```python
from build123d import *

# Parameters (mm, degrees)
F0_R     = 30.180652
F1_DEPTH = 254
F2_R     = 23.830652
F3_DEPTH = 102.916548
F4_R     = 5.08
F6_W     = 42.340428
F6_H     = 35.694406
F7_DEPTH = 45.834139


with BuildPart() as f1:
    # F0 (on Top) → F1 (new body)
    with BuildSketch(Plane.XY):
        Circle(F0_R)
    extrude(amount=-F1_DEPTH)

    # F2 (on face) → F3 (cut)
    with BuildSketch(Plane(origin=(0, 0, -254), x_dir=(1, 0, 0), z_dir=(0, 0, -1))):
        Circle(F2_R)
    extrude(amount=-F3_DEPTH, mode=Mode.SUBTRACT)

    # F4
    f4_edges = [f1.edges().sort_by_distance(p)[0] for p in [
        (30.180652, 0, -127),
        (-30.180652, 0, 0),
        (-30.180652, 0, -254),
    ]]
    fillet(f4_edges, radius=F4_R)

    # F6 (on offset) → F7 (join)
    with BuildSketch(Plane.YZ.offset(55.124739)):
        with Locations((3.907934, -50.849177)):
            Rectangle(F6_W, F6_H)
    extrude(amount=-F7_DEPTH)


solid = f1.part
```
For this review, take the finished solid that the model builds, in its own axes (mm). A direction names the side the tool comes from. Round coordinates to 2 decimals unless told otherwise and drop trailing zeros. Write each loop counter-clockwise with the first axis right and the second up, starting at its lowest first coordinate (ties: lowest second). Pieces come first, ordered by that corner, then holes.
1) Take a section at B-B on y = 0. Give the boundary of the cut face in (x, z), then the cut area to 3 significant figures.
Answer below:
outline: (-30.18, -248.92) arc R5.08 ccw to (-25.1, -254) - (-23.83, -254) - (-23.83, -151.08) - (23.83, -151.08) - (23.83, -254) - (25.1, -254) arc R5.08 ccw to (30.18, -248.92) - (30.18, -68.7) - (55.12, -68.7) - (55.12, -33) - (30.18, -33) - (30.18, -5.08) arc R5.08 ccw to (25.1, 0) - (-25.1, 0) arc R5.08 ccw to (-30.18, -5.08) - close
area: 11,300 mm2
2) For line 1 along Y through (x, z) = (0, -228); line 2 along Z through (x, y) = (12.5, -9); line 3 along Y through (x, z) = (2.5, -242.5), list the stretches that pass through material, from the lowest coordinate up.
Answer below:
line 1: y = -30.18 to -23.83, 23.83 to 30.18
line 2: z = -151.08 to 0
line 3: y = -30.08 to -23.7, 23.7 to 30.08
3) Take a section at A-A on x = 0. Give the boundary of the cut face in (y, z), then the cut area to 3 significant figures.
Answer below:
outline: (-30.18, -248.92) arc R5.08 ccw to (-25.1, -254) - (-23.83, -254) - (-23.83, -151.08) - (23.83, -151.08) - (23.83, -254) - (25.1, -254) arc R5.08 ccw to (30.18, -248.92) - (30.18, -5.08) arc R5.08 ccw to (25.1, 0) - (-25.1, 0) arc R5.08 ccw to (-30.18, -5.08) - close
area: 10,400 mm2
4) Machinability: for faces 1 (the face through (12.8, -20.1, -203.3)), 2 (the face through (22.2, -9.2, -254)), 3 (the face through (40, -17.262, -51)), which of the approach directions +Z, -Z, +X, -X, +Y, -Y give a long, thin tool a straight path to every point of the face, cutting with its end or side? Answer none if there is none.
Answer below:
face 1: -Z
face 2: -Z, +X, -X, +Y, -Y
face 3: +Z, -Z, +X, -Y
5) Take a section at D-D on x = 40. Give the boundary of the cut face in (y, z), then the cut area to 3 significant figures.
Answer below:
outline: (-17.26, -68.7) - (25.08, -68.7) - (25.08, -33) - (-17.26, -33) - close
area: 1,510 mm2
6) Mouldability with a two-part tool opening along Y and no side actions: class faces 4 (the face through (0, 0, -151.083)), 5 (the face through (0, 0, 0)), 6 (the face through (36, 25.078, -51)) as +Y half, -Y half, draft (parallel to the pull), parting line (faces both ways), or undercut.
Answer below:
face 4: undercut
face 5: draft
face 6: +Y half
7) Take a section at C-C on z = -42. Give the boundary of the cut face in (x, y), then the cut area to 3 significant figures.
Answer below:
outline: (16.79, 25.08) arc R30.18 ccw (long way) to (24.76, -17.26) - (55.12, -17.26) - (55.12, 25.08) - close
area: 4,050 mm2
8) Insertion check: pin 1 Ø10 at (x, y) = (8, -0.5) entering from +Z; pin 2 Ø15 at (x, z) = (46, -55) entering from -Y; pin 3 Ø6 at (x, y) = (-6, 6) entering from -Z; pin 4 Ø2 at (x, z) = (5, -167.5) entering from +Y. Each pin has a flat end and moves straight along its axis. Give the tip position at first contact, or say it passes through.
Answer below:
pin 1: stops at z = 0
pin 2: stops at y = -17.26
pin 3: stops at z = -151.08
pin 4: stops at y = 29.91
